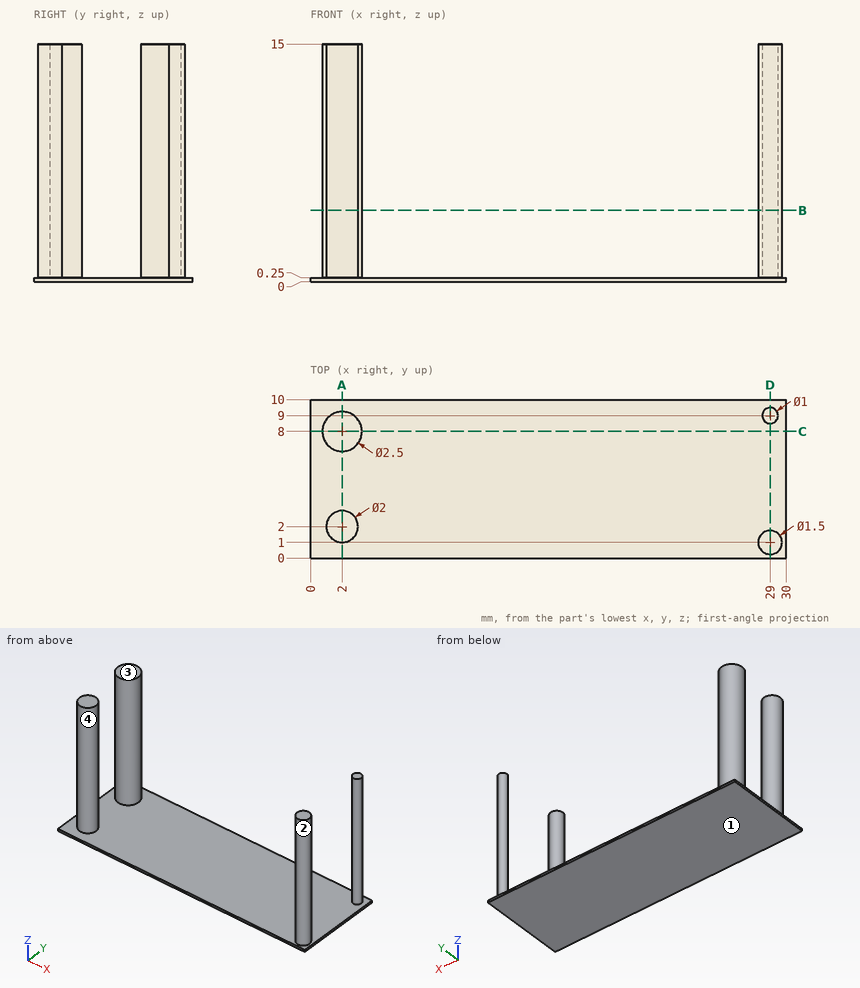
Verification items for this drawing (mm, ordinates from the low corner). A direction names the side the tool comes from. Coordinates: 2 decimals unless noted, no trailing zeros. Loops run counter-clockwise (first coordinate to the right, second up) from the corner with the lowest first, then second, coordinate; pieces in that order, holes last.
Item 1: Sectioned sample at C-C, the plane y = 8. Record the boundary of the cut face in (x, z), then the cut area to 3 significant figures.
Item 2: Access from +Z, -Z, +X, -X, +Y, -Y to the whole of each face (thin tool, end or side, straight path). Record for the marked faces 1 and 2.
Item 3: Go/stop test with flat-tipped pins: pin 1 Ø3 at (y, z) = (3.5, 10.5) entering from -X; pin 2 Ø5 at (x, y) = (16.5, 3.5) entering from +Z. Record where each tip stops, or that it passes through.
Item 4: Sectioned sample at D-D, the plane x = 29. Record the boundary of the cut face in (y, z), then the cut area to 3 significant figures.
Item 5: Release check for a two-part mould opening along Y. For the marked faces 3 and 4 record: released by +Y, released by -Y, zero draft, split by the parting line, or undercut.
Item 6: Thickness scan on line 1 (Z direction, x = 7.5, y = 8.5); line 2 (X direction, y = 8.25, z = 1); line 3 (Y direction, x = 28.75, z = 2.75). Record the ranges inside material, lowest first.
Item 7: Sectioned sample at A-A, the plane x = 2. Record the boundary of the cut face in (y, z), then the cut area to 3 significant figures.
Item 8: Sectioned sample at B-B, the plane z = 4.5. Record the boundary of the cut face in (x, y).
Check result:
1. outline: (0, 0) - (30, 0) - (30, 0.25) - (3.25, 0.25) - (3.25, 15) - (0.75, 15) - (0.75, 0.25) - (0, 0.25) - close
1. area: 44.4 mm2
2. face 1: -Z, +X, -X, +Y, -Y
2. face 2: +Z
3. pin 1: stops at x = 1
3. pin 2: stops at z = 0.25
4. outline: (0, 0) - (10, 0) - (10, 0.25) - (9.5, 0.25) - (9.5, 15) - (8.5, 15) - (8.5, 0.25) - (1.75, 0.25) - (1.75, 15) - (0.25, 15) - (0.25, 0.25) - (0, 0.25) - close
4. area: 39.4 mm2
5. face 3: zero draft
5. face 4: undercut
6. line 1: z = 0 to 0.25
6. line 2: x = 0.78 to 3.22
6. line 3: y = 0.29 to 1.71, 8.57 to 9.43
7. outline: (0, 0) - (10, 0) - (10, 0.25) - (9.25, 0.25) - (9.25, 15) - (6.75, 15) - (6.75, 0.25) - (3, 0.25) - (3, 15) - (1, 15) - (1, 0.25) - (0, 0.25) - close
7. area: 68.9 mm2
8. outline: circle Ø2.5 at (2, 8); circle Ø2 at (2, 2); circle Ø1.5 at (29, 1); circle Ø1 at (29, 9)
